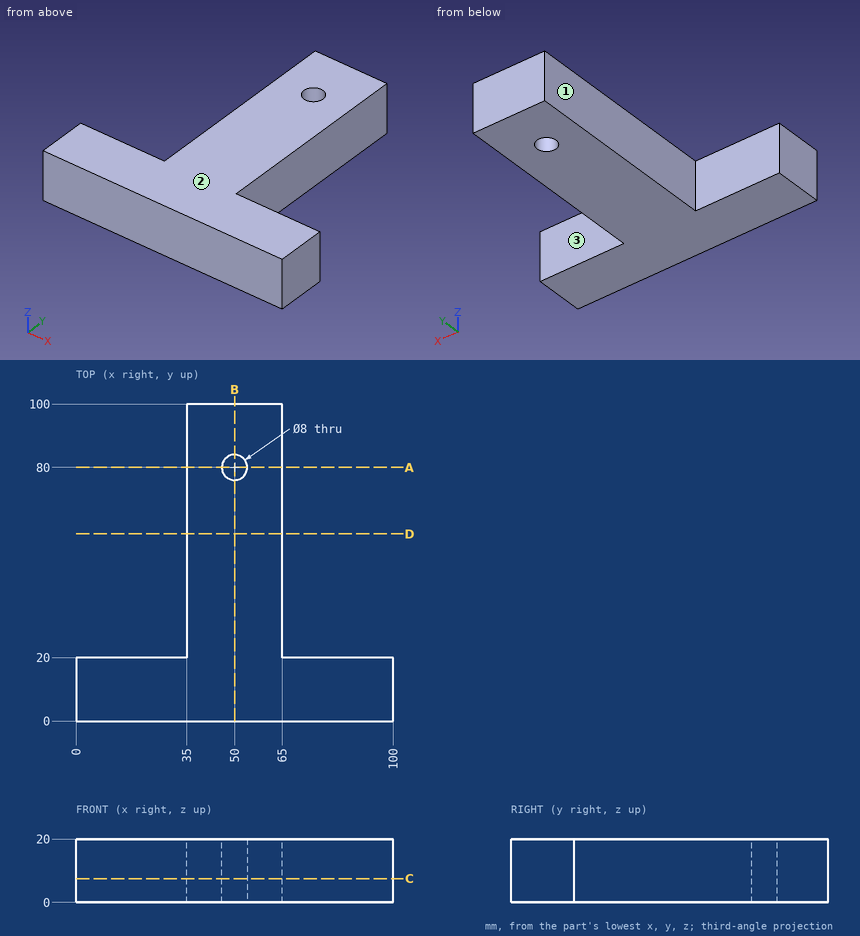
For this review, use the dimensioned drawing (mm, ordinates from the lowest corner) and the shaded views. A direction names the side the tool comes from. Round coordinates to 2 decimals unless told otherwise and drop trailing zeros. Write each loop counter-clockwise with the first axis right and the second up, starting at its lowest first coordinate (ties: lowest second). Pieces come first, ordered by that corner, then holes. Notation, with made-up numbers: (47.25, 37.5) - (98.25, 37.5) arc R26 ccw to (98.25, 75.5) - close; hole circle Ø8 at (13, 81). An arc over 180 degrees is marked (long way). One line per item, written item: value. Start each with the question number.
1. Consider section D-D on y = 59. Write out the cut boundary in (x, z).
2. Machinability: for the marked faces 1, 2 and 3, which of the approach directions +Z, -Z, +X, -X, +Y, -Y give a long, thin tool a straight path to every point of the face, cutting with its end or side? Answer none if there is none.
3. Consider section A-A on y = 80. Write out the cut boundary in (x, z), and give its area (3 significant figures).
4. Consider section B-B on x = 50. Write out the cut boundary in (y, z).
5. Consider section C-C on z = 7.5. Write out the cut boundary in (x, y), and give its area (3 significant figures).
6. Clearance check with flat-ended pins moving along their axes: P1, Ø5, axis at y = 63.5, z = 18, coming from the -X side; P2, Ø1.5, axis at y = 63, z = 7, coming from the +X side; P3, Ø6, axis at x = 88, z = 10, coming from the +Y side. State where each tip first meets the part, or that it passes through.
7. To check wall thickness, follow L1, parallel to Y at x = 50, z = 12.5; L2, parallel to X at y = 29, z = 9.75; L3, parallel to Y at x = 26.5, z = 6. State the ranges of each line that lie inside material, in increasing order. Write a range as from..to.
Checks:
1. outline: (35, 0) - (65, 0) - (65, 20) - (35, 20) - close
2. face 1: +Z, -Z, -X, +Y
2. face 2: +Z, +X, -X, +Y, -Y
2. face 3: +Z, -Z, +X, +Y
3. outline: (35, 0) - (46, 0) - (46, 20) - (35, 20) - close; (54, 0) - (65, 0) - (65, 20) - (54, 20) - close
3. area: 440 mm^2
4. outline: (0, 0) - (76, 0) - (76, 20) - (0, 20) - close; (84, 0) - (100, 0) - (100, 20) - (84, 20) - close
5. outline: (0, 0) - (100, 0) - (100, 20) - (65, 20) - (65, 100) - (35, 100) - (35, 20) - (0, 20) - close; hole circle Ø8 at (50, 80)
5. area: 4,350 mm^2
6. P1: stops at x = 35
6. P2: stops at x = 65
6. P3: stops at y = 20
7. L1: y = 0..76, 84..100
7. L2: x = 35..65
7. L3: y = 0..20
